from build123d import *

# Parameters (mm, degrees)
F0_R     = 1.325
F1_DEPTH = 1.6


with BuildPart() as f1:
    # F0 (on Top) → F1 (new body)
    with BuildSketch(Plane.XY):
        Polygon((0, 10), (0, 0), (24.125, 0), (55.875, 0), (80, 0), (80, 10), (55.875, 10), (24.125, 10), align=None)
        with Locations((28.09375, 7.46)):
            Circle(F0_R, mode=Mode.SUBTRACT)
        with BuildLine():
            ThreePointArc((53.23125, 7.46), (51.90625, 6.135), (50.58125, 7.46))
            ThreePointArc((50.58125, 7.46), (51.90625, 8.785), (53.23125, 7.46))
        make_face(mode=Mode.SUBTRACT)
    extrude(amount=F1_DEPTH)


solid = f1.part
Here's how the part is built. I have some questions about the finished solid (model axes, mm). Coordinates: 2 decimals unless noted, no trailing zeros. Order: outer loops, then holes, each group sorted by start corner. A loop starts at its lowest first (then second) coordinate and runs counter-clockwise, first axis right, second up.
Item 1: If we section it at A-A on y = 7.46: List the corners of the cut face in (x, z) for me.
Result sheet:
outline: (0, 0) - (26.77, 0) - (26.77, 1.6) - (0, 1.6) - close; (29.42, 0) - (50.58, 0) - (50.58, 1.6) - (29.42, 1.6) - close; (53.23, 0) - (80, 0) - (80, 1.6) - (53.23, 1.6) - close
Item 2: I need wall thicknesses on line 1 (Y direction, x = 28, z = 0.25); line 2 (X direction, y = 8, z = 0.1); line 3 (X direction, y = 8.5, z = 0.3). Which ranges of each line are inside material? Lowest first, please.
Result sheet:
line 1: y = 0 to 6.14, 8.78 to 10
line 2: x = 0 to 26.88, 29.3 to 50.7, 53.12 to 80
line 3: x = 0 to 27.27, 28.91 to 51.09, 52.73 to 80
Item 3: If we mould it in two halves opening along Y, with no side actions, what happens to faces 1 (the face through (52.079, 8.774, 0.789)), 2 (the face through (39, 5, 1.6)), 3 (the face through (41, 10, 1))? For each: +Y half, -Y half, draft (parallel to the pull), parting line (faces both ways), or undercut.
Result sheet:
face 1: undercut
face 2: draft
face 3: +Y half
